Build history of the part. All positions in model axes, mm. Face numbers are marked on the shaded views. Round coordinates to 2 decimals unless told otherwise and drop trailing zeros. Write each loop counter-clockwise with the first axis right and the second up, starting at its lowest first coordinate (ties: lowest second). Pieces come first, ordered by that corner, then holes. Notation, with made-up numbers: M 21,48 L 47,48 A17 ccw 47,62 Z; hole C -12,76.5 d2. An arc over 180 degrees is marked long. Write item = value, one per line. Start each with the question number.
Q1. Band-saw the part on D-D on y = 0. Write the cut outline in (x, z).
Q2. Pull direction X, two halves, no side cores. Call the marked faces 1 and 2: released by +X, released by -X, zero draft, split by the parting line, or undercut.
Q3. Band-saw the part on A-A on x = 7.25. Write the cut outline in (y, z).
Q4. Band-saw the part on B-B on y = -0.75. Write the cut outline in (x, z), plus the area to 3 significant figures.
Q5. Band-saw the part on C-C on z = 1.75. Write the cut outline in (x, y), plus the area to 3 significant figures.
Q6. Drop a flat-ended pin along its axis: P1, Ø2, axis at x = -3.5, y = -1.5, coming from the +Z side. Give the stop position or say it passes through.
Q7. Probe L1, parallel to Z at x = 8.75, y = 1.5; L2, parallel to X at y = 0.5, z = 1.6. List the from-to ranges inside material, lowest first.
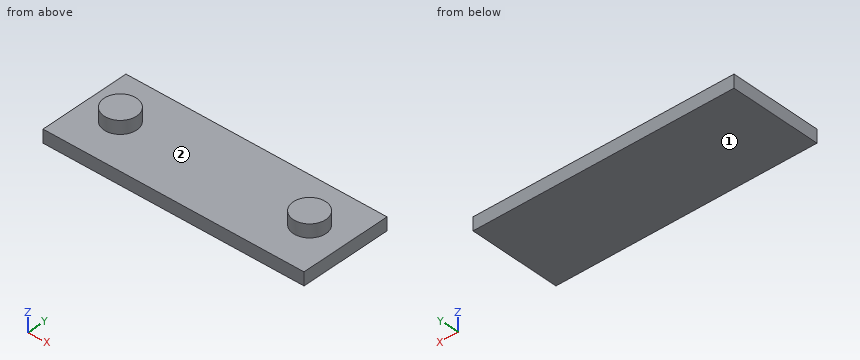
```python
from build123d import *

# Parameters (mm, degrees)
SKETCH1_W           = 20
SKETCH1_H           = 7
BOSS_EXTRUDE1_DEPTH = 1
SKETCH2_R           = 1.25
BOSS_EXTRUDE2_DEPTH = 1


with BuildPart() as part:
    # Sketch1 → Boss-Extrude1 (new body)
    with BuildSketch(Plane.XY):
        Rectangle(SKETCH1_W, SKETCH1_H)
    extrude(amount=BOSS_EXTRUDE1_DEPTH)

    # Sketch2 → Boss-Extrude2 (add)
    with BuildSketch(Plane.XY.offset(1)):
        with Locations((-7.25, 0)):
            Circle(SKETCH2_R)
        with Locations((7.25, 0)):
            Circle(SKETCH2_R)
    extrude(amount=BOSS_EXTRUDE2_DEPTH)


solid = part.part
```
Conclusion:
q1.outline = M -10,0 L 10,0 L 10,1 L 8.5,1 L 8.5,2 L 6,2 L 6,1 L -6,1 L -6,2 L -8.5,2 L -8.5,1 L -10,1 Z
q2.face_1 = zero draft
q2.face_2 = undercut
q3.outline = M -3.5,0 L 3.5,0 L 3.5,1 L 1.25,1 L 1.25,2 L -1.25,2 L -1.25,1 L -3.5,1 Z
q4.outline = M -10,0 L 10,0 L 10,1 L 8.25,1 L 8.25,2 L 6.25,2 L 6.25,1 L -6.25,1 L -6.25,2 L -8.25,2 L -8.25,1 L -10,1 Z
q4.area = 24.0 mm^2
q5.outline = C -7.25,0 d2.5; C 7.25,0 d2.5
q5.area = 9.82 mm^2
q6.P1 = 1
q7.L1 = 0 to 1
q7.L2 = -8.4 to -6.1, 6.1 to 8.4
